from build123d import *

# Parameters (mm, degrees)
FILLET1_R    = 0.6
RECPAT_COUNT = 2
RECPAT_ANGLE = 90


with BuildPart() as part:
    # BodySke → BaseBody (revolve)
    with BuildSketch(Plane.XY, mode=Mode.PRIVATE) as basebody_sk:
        with BuildLine():
            Line((6, 4), (6, 8))
            Line((6, 8), (2.753049234, 8))
            ThreePointArc((2.753049234, 8), (0.707515305, 4.230226947), (0, 0))
            Line((0, 0), (56, 0))
            Line((56, 0), (56, 4))
            Line((56, 4), (6, 4))
        make_face()
    revolve(basebody_sk.sketch.rotate(Axis((0, 0, 0), (1, 0, 0)), 90), axis=Axis((0, 0, 0), (1, 0, 0)))

    # Fillet1
    fillet1_edges = [part.edges().sort_by_distance(p)[0] for p in [
        (6, 0, -4),
    ]]
    fillet(fillet1_edges, radius=FILLET1_R)

    # RecSkeTop → Recess section 0
    with BuildSketch(Plane(origin=(0, 0, 0), x_dir=(0, 0, -1), z_dir=(1, 0, 0))):
        with BuildLine():
            Line((-0.968, 4.4), (0.968, 4.4))
            Line((0.968, 4.4), (0.968, -4.4))
            Line((0.968, -4.4), (-0.968, -4.4))
            Line((-0.968, -4.4), (-0.968, 4.4))
        make_face()
    # RecSkeBot → Recess section 1
    with BuildSketch(Plane(origin=(4.5, 0, 0), x_dir=(0, 0, -1), z_dir=(1, 0, 0))):
        with BuildLine():
            Line((-0.968, 2.156383139), (0.968, 2.156383139))
            Line((0.968, 2.156383139), (0.968, -2.156383139))
            Line((0.968, -2.156383139), (-0.968, -2.156383139))
            Line((-0.968, -2.156383139), (-0.968, 2.156383139))
        make_face()
    recess = loft(mode=Mode.SUBTRACT)

    # RecPat: Recess ×2 about axis
    recpat_axis = Axis((0, 0, 0), (1, 0, 0))
    for i in range(1, RECPAT_COUNT):
        add(recess.rotate(recpat_axis, i * RECPAT_ANGLE / (RECPAT_COUNT - 1)), mode=Mode.SUBTRACT)

    # RecCorSke → RecessCore (revolve, cut)
    with BuildSketch(Plane.XY, mode=Mode.PRIVATE) as recesscore_sk:
        Polygon((0, 0), (0, 2.1296), (4.5, 1.814929346), (5.089706292, 0), align=None)
    revolve(recesscore_sk.sketch.rotate(Axis((0, 0, 0), (1, 0, 0)), 346.581092025), axis=Axis((0, 0, 0), (1, 0, 0)), mode=Mode.SUBTRACT)


solid = part.part
Geometry: final body of the model. Coordinates: model frame, mm. A direction names the side the tool comes from. Give positions to 0.01 mm unless a question says otherwise; leave off trailing zeros. Loops run counter-clockwise (first coordinate to the right, second up) from the corner with the lowest first, then second, coordinate; pieces in that order, holes last. Notation, with made-up numbers: (71.5, 54) - (97.5, 54) arc R10 cw to (97.5, 68) - close; hole circle Ø4 at (-16.75, 65). An arc over 180 degrees is marked (long way). One line per question, with ' | ' between items. Start each with the question number.
(1) Reachability of faces 4 (the conical face through (2.367, 1.383, -1.395)), 5 (the flat face through (6, 3.4, -3.4)), 6 (the cylindrical face through (4.35, 7.81, -1.73)) from +Z, -Z, +X, -X, +Y, -Y: full face, straight path, thin tool, end or side. Return the list, or none.
(2) Section query C-C on z = 6. Return loops of the section in (x, y).
(3) Section query A-A on x = 18.5. Return loops of the section in (y, z).
(4) Pull-direction query (Y, two-part tool) for faces 1 (the flat face through (56, 0, 0)), 2 (the cylindrical face through (30.954, 3.905, -0.867)), 3 (the conical face through (2.367, -1.383, 1.395)); classes: released by +Y, released by -Y, zero draft, split by the parting line, or undercut.
(5) Ray query, line 1 (Z direction, x = 7.5, y = -2.75); line 2 (Y direction, x = 54.5, z = 1.5); line 3 (X direction, y = 6.75, z = 3.75). Return the intervals inside material, ascending. Write a range as from..to.
(6) Contact query for flat-ended pins moving along their axis: pin 1 (1.5 mm diameter, centred on x = 8, y = -5.5, fed in from +Z); pin 2 (5 mm diameter, centred on y = -1, z = 4, fed in from -X); pin 3 (4 mm diameter, centred on x = 49.5, z = 2.5, fed in from -Y); pin 4 (1 mm diameter, centred on x = 11.5, z = -1.5, fed in from -Y). Output: stop coordinate, or through.
(7) Section query B-B on y = 5.75. Return loops of the section in (x, z).
The answers:
1) face 4: -X | face 5: +X | face 6: +X, -X
2) outline: (2.75, -5.29) - (6, -5.29) - (6, 5.29) - (2.75, 5.29) arc R11.53 ccw to start
3) outline: circle Ø8 at (0, 0)
4) face 1: zero draft | face 2: split by the parting line | face 3: undercut
5) line 1: -2.9..2.9 | line 2: -3.71..3.71 | line 3: 2.54..6
6) pin 1: through | pin 2: x = 0.17 | pin 3: y = -3.97 | pin 4: y = -3.87
7) outline: (2.75, -5.56) - (6, -5.56) - (6, 5.56) - (2.75, 5.56) arc R11.66 ccw to start
